Geometry: final body of the model. Coordinates: model frame, mm. A direction names the side the tool comes from. Coordinates: 2 decimals unless noted, no trailing zeros. Loops run counter-clockwise (first coordinate to the right, second up) from the corner with the lowest first, then second, coordinate; pieces in that order, holes last. Notation, with made-up numbers: (-4, 84) - (44, 84) arc R38 cw to (44, 122) - close; hole circle Ø2 at (54, 34). An arc over 180 degrees is marked (long way). Return JSON: item names as keys, results as strings.
Autodesk Inventor part; units mm, degrees
ref_plane "YZ Plane" through (0, 0, 0) normal (1, 0, 0) x (0, 1, 0)
ref_plane "XZ Plane" through (0, 0, 0) normal (0, 1, 0) x (-1, 0, 0)
ref_plane "XY Plane" through (0, 0, 0) normal (0, 0, 1) x (1, 0, 0)
sketch "Sketch1" plane through (0, 0, 0) normal (0, 1, 0) x (-1, 0, 0)
  line L0 (0, 0) -> (-40.386, 0)
  line L1 (-40.386, 0) -> (-40.386, -50.165)
  line L2 (-40.386, -50.165) -> (0, -50.165)
  circle A0 centre (-8.636, -12.446) radius 7.366
  line L3 (-1.27, -45.085) -> (-1.27, -30.353)
  line L4 (-1.27, -30.353) -> (-16.002, -30.353)
  line L5 (-16.002, -30.353) -> (-16.002, -45.085)
  line L6 (-16.002, -45.085) -> (-1.27, -45.085)
  line L7 (-31.0134, -45.085) -> (-22.9108, -31.0509)
  line L8 (-22.9108, -31.0509) -> (-39.116, -31.0509)
  line L9 (-39.116, -31.0509) -> (-31.0134, -45.085)
  line L10 (-40.386, 0) -> (-40.386, -12.3952)
  line L11 (-38.8493, -12.3952) -> (-35.3989, -15.4707)
  line L12 (-33.5401, -19.7026) -> (-35.3989, -15.4707)
  line L13 (-24.9497, -7.879) -> (-25.9334, -12.3952)
  line L14 (-24.9497, -16.9114) -> (-25.9334, -12.3952)
  line L15 (-24.9497, -16.9114) -> (-29.2449, -17.2623)
  line L16 (-33.5401, -19.7026) -> (-29.2449, -17.2623)
  line L17 (-33.5401, -5.0878) -> (-29.2449, -7.5281)
  line L18 (-24.9497, -7.879) -> (-29.2449, -7.5281)
  line L19 (-38.8493, -12.3952) -> (-35.3989, -9.3197)
  line L20 (-33.5401, -5.0878) -> (-35.3989, -9.3197)
  line L21 (0, -50.165) -> (0, 0)
  point P0 (-31.1658, -12.3952)
  dimension "d0" = 40.386
  dimension "d1" = 50.165
  dimension "d4" = 14.732
  dimension "d7" = 14.732
  dimension "d8" = 14.732
  dimension "d15" = 12.3952
extrude "Extrusion1" add sketch "Sketch1" along normal blind 7.62
fillet "Fillet1" radius 5.08 4 edges at (40.386, 3.81, 0) (40.386, 3.81, -50.165) (0, 3.81, -50.165) (0, 3.81, 0)
shell "Shell1" thickness 0.254 removed faces 1 at (23.3087, 0, -40.407)
properties part number "PassengerBaseGBR"
Item 1: Ray query, probe 1 along X at (y, z) = (2.5, -24); probe 2 along Z at (x, y) = (14, 3.75) (3 decimals); probe 3 along X at (y, z) = (4, -41). Return the intervals inside material, ascending. Write a range as from..to.
Worked out:
{"probe 1": "0..0.25, 40.13..40.39", "probe 2": "-50.165..-49.911, -45.339..-45.085, -30.353..-30.099, -17.858..-17.494, -7.398..-7.034, -0.254..0", "probe 3": "0..0.25, 1.02..1.27, 16..16.26, 28.36..28.65, 33.37..33.67, 40.13..40.39"}
Item 2: Section query A-A, the plane x = 17.5. Return loops of the section in (y, z) (3 decimals), and give its area (3 significant figures).
Worked out:
{"outline": "(0, -50.165) - (7.62, -50.165) - (7.62, 0) - (0, 0) - (0, -0.254) - (7.366, -0.254) - (7.366, -49.911) - (0, -49.911) - close", "area": "16.5 mm^2"}
Item 3: Section query C-C, the plane x = 8.5. Return loops of the section in (y, z) (3 decimals), and give its area (3 significant figures).
Worked out:
{"outline": "(0, -50.165) - (7.62, -50.165) - (7.62, -45.085) - (0, -45.085) - (0, -45.339) - (7.366, -45.339) - (7.366, -49.911) - (0, -49.911) - close; (0, -30.353) - (7.62, -30.353) - (7.62, -19.811) - (0, -19.811) - (0, -20.065) - (7.366, -20.065) - (7.366, -30.099) - (0, -30.099) - close; (0, -5.081) - (7.62, -5.081) - (7.62, 0) - (0, 0) - (0, -0.254) - (7.366, -0.254) - (7.366, -4.827) - (0, -4.827) - close", "area": "16.5 mm^2"}
Item 4: First-contact query: pin 1 Ø8 at (x, z) = (24.5, -11.5) entering from -Y; pin 2 Ø12 at (x, z) = (8.636, -12.446) entering from +Y. Flat tips, straight axial feed; report the tip coordinate or a pass-through.
Worked out:
{"pin 1": "y = 0", "pin 2": "through"}
Item 5: Section query B-B, the plane z = -32. Return loops of the section in (x, y).
Worked out:
{"outline": "(0, 0) - (0.25, 0) - (0.25, 7.37) - (1.02, 7.37) - (1.02, 0) - (1.27, 0) - (1.27, 7.62) - (0, 7.62) - close; (16, 0) - (16.26, 0) - (16.26, 7.37) - (23.17, 7.37) - (23.17, 0) - (23.46, 0) - (23.46, 7.62) - (16, 7.62) - close; (38.57, 0) - (38.86, 0) - (38.86, 7.37) - (40.13, 7.37) - (40.13, 0) - (40.39, 0) - (40.39, 7.62) - (38.57, 7.62) - close"}
Item 6: Mould query, pull axis Z, two halves, no side actions, for faces 4 (the face through (0, 4, -25)), 5 (the face through (38.86, 3.86, -1.45)), 6 (the face through (35.12, 3.76, -37.97)). Classes: +Z half, -Z half, draft (parallel to the pull), parting line (faces both ways), or undercut.
Worked out:
{"face 4": "draft", "face 5": "+Z half", "face 6": "undercut"}
Item 7: Reachability of faces 1 (the face through (38.68, 3.73, -1.63)), 2 (the face through (37.15, 3.76, -10.88)), 3 (the face through (40.386, 4, -25)) from +Z, -Z, +X, -X, +Y, -Y: full face, straight path, thin tool, end or side. Return the list, or none.
Worked out:
{"face 1": "-Y", "face 2": "+Y, -Y", "face 3": "+Z, -Z, +X, +Y, -Y"}
Item 8: Section query D-D, the plane z = -2.5. Return loops of the section in (x, y).
Worked out:
{"outline": "(0.7, 0) - (1, 0) - (1, 7.37) - (39.38, 7.37) - (39.38, 0) - (39.68, 0) - (39.68, 7.62) - (0.7, 7.62) - close"}
